from build123d import *

# Parameters (mm, degrees)
SCHIZZO1_W                   = 335
SCHIZZO1_H                   = 50
SCHIZZO1_R                   = 7.5
SCHIZZO1_R_2                 = 10
ESTRUSIONE_ESTRUSIONE1_DEPTH = 5
SCHIZZO2_R                   = 2.75
TAGLIO_ESTRUSIONE1_DEPTH     = 297.226264872
RIPETIZIONECIRCOLARE1_COUNT  = 8
RACCORDO1_R                  = 25
SCHIZZO3_R                   = 2.1
TAGLIO_ESTRUSIONE2_DEPTH     = 297.226264872
SCHIZZO4_R                   = 21
TAGLIO_ESTRUSIONE3_DEPTH     = 3
SMUSSO1_SIZE                 = 0.5


with BuildPart() as part:
    # Schizzo1 → Estrusione-Estrusione1 (new, symmetric)
    with BuildSketch(Plane(origin=(0, 0, 0), x_dir=(1, 0, 0), z_dir=(0, 1, 0))):
        with Locations((-127.5, 0)):
            Rectangle(SCHIZZO1_W, SCHIZZO1_H)
        with Locations(Location((0, 0, 0), (0, 0, 270))):
            Circle(SCHIZZO1_R, mode=Mode.SUBTRACT)
        with Locations(Location((-260, 0, 0), (0, 0, 270))):
            Circle(SCHIZZO1_R_2, mode=Mode.SUBTRACT)
    extrude(amount=ESTRUSIONE_ESTRUSIONE1_DEPTH, both=True)

    # Schizzo2 → Taglio-Estrusione1 (cut, through all)
    with BuildSketch(Plane(origin=(0, 5, 0), x_dir=(1, 0, 0), z_dir=(0, 1, 0))):
        with Locations(Location((-16, 0, 0), (0, 0, 270))):
            Circle(SCHIZZO2_R)
    taglio_estrusione1 = extrude(amount=-TAGLIO_ESTRUSIONE1_DEPTH, mode=Mode.SUBTRACT)

    # RipetizioneCircolare1: Taglio-Estrusione1 ×8 about axis
    ripetizionecircolare1_axis = Axis((0, 0, 0), (0, 1, 0))
    for i in range(1, RIPETIZIONECIRCOLARE1_COUNT):
        add(taglio_estrusione1.rotate(ripetizionecircolare1_axis, i * 360 / RIPETIZIONECIRCOLARE1_COUNT), mode=Mode.SUBTRACT)

    # Raccordo1
    raccordo1_edges = [part.edges().sort_by_distance(p)[0] for p in [
        (40, 0, 25),
        (40, 0, -25),
    ]]
    fillet(raccordo1_edges, radius=RACCORDO1_R - 0.0001)  # a hair under: the kernel refuses the full size

    # Schizzo3 → Taglio-Estrusione2 (cut, through all)
    with BuildSketch(Plane(origin=(0, 5, 0), x_dir=(1, 0, 0), z_dir=(0, 1, 0))):
        with Locations(Location((-100, 0, 0), (0, 0, 270))):
            Circle(SCHIZZO3_R)
    extrude(amount=-TAGLIO_ESTRUSIONE2_DEPTH, mode=Mode.SUBTRACT)

    # Schizzo4 → Taglio-Estrusione3 (cut)
    with BuildSketch(Plane.XZ.offset(5)):
        with Locations(Location((0, 0, 0), (0, 0, 270))):
            Circle(SCHIZZO4_R)
    extrude(amount=-TAGLIO_ESTRUSIONE3_DEPTH, mode=Mode.SUBTRACT)

    # Smusso1
    smusso1_edges = [part.edges().sort_by_distance(p)[0] for p in [
        (0, -5, 21),
    ]]
    chamfer(smusso1_edges, length=SMUSSO1_SIZE)


solid = part.part
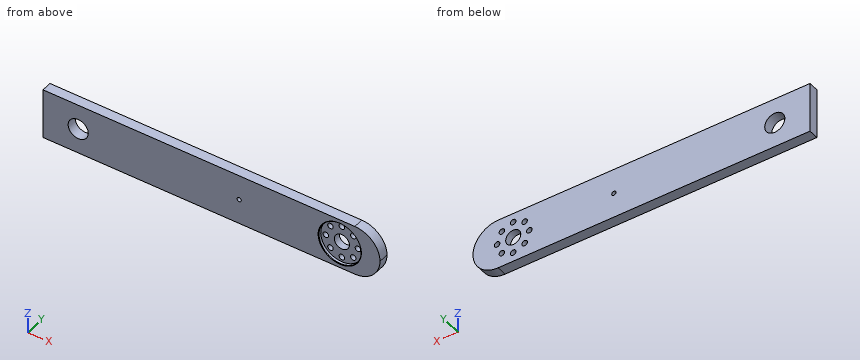
Verification items for the finished model (mm, model axes). Coordinates: 2 decimals unless noted, no trailing zeros. Write each loop counter-clockwise with the first axis right and the second up, starting at its lowest first coordinate (ties: lowest second). Pieces come first, ordered by that corner, then holes. Notation, with made-up numbers: (-12.5, 19) -> (-4.5, 19) arc R21 ccw to (-4.5, 58) -> close; hole circle Ø8 at (25, 68.25). An arc over 180 degrees is marked (long way). One line per item, written item: value. Start each with the question number.
Q1. Cross-section at B-B on y = 2. State how many separate pieces and enclosed holes the cut face has, and give its area (3 significant figures).
Q2. Thickness scan on L1, parallel to Z at x = 0, y = 2.75; L2, parallel to X at y = -0.25, z = 0; L3, parallel to Z at x = 2, y = 4. Record the ranges inside material, lowest first. Write a range as from..to.
Q3. Go/stop test with flat-tipped pins: P1, Ø12.5, axis at x = 7.5, z = -7.5, coming from the -Y side; P2, Ø6.5, axis at x = 11.31, z = -11.31, coming from the +Y side; P3, Ø3.5, axis at x = -11.31, z = -11.31, coming from the +Y side; P4, Ø1.5, axis at y = 2, z = 5.5, coming from the +X side. Record where each tip stops, or that it passes through.
Q4. Cross-section at A-A on x = -260. Enter the section's corners in (y, z), and give its area (3 significant figures).
Checked values:
1. separate pieces: 1
1. enclosed holes: 11
1. area: 15,800 mm²
2. L1: z = -25..-18.75, -13.25..-7.5, 7.5..13.25, 18.75..25
2. L2: x = -295..-270, -250..-102.1, -97.9..-18.75, -13.25..-7.5, 7.5..13.25, 18.75..40
2. L3: z = -25..-17.89, -14.11..-7.23, 7.23..14.11, 17.89..25
3. P1: stops at y = -2
3. P2: stops at y = 5
3. P3: passes through
3. P4: stops at x = 39.54
4. outline: (-5, -25) -> (5, -25) -> (5, -10) -> (-5, -10) -> close; (-5, 10) -> (5, 10) -> (5, 25) -> (-5, 25) -> close
4. area: 300 mm²
